The listing builds one solid part. Answer for the finished solid, in the listing's coordinates (mm). A direction names the side the tool comes from. Coordinates: 2 decimals unless noted, no trailing zeros. Loops run counter-clockwise (first coordinate to the right, second up) from the corner with the lowest first, then second, coordinate; pieces in that order, holes last. Notation, with made-up numbers: (-12.5, -31.5) - (16.5, -31.5) arc R31 ccw to (16.5, -5.5) - close; hole circle Ø7 at (78, -17). An arc over 180 degrees is marked (long way). Return JSON: item names as keys, results as strings. Group by question number.
1. Which of the six approach directions +Z, -Z, +X, -X, +Y, -Y give full straight-line access (tool end or side, diameter ignored) to faces 4 (the face through (0, 0.65, 1.4)), 5 (the face through (0.19, 7.45, 0.87)), 6 (the face through (-0.19, -7.49, 0.87))?
2. Each of these flat-tipped pins is pushed along its axis until it touches: P1, Ø1.5, axis at x = 1.5, y = 1, coming from the -Z side; P2, Ø1.6, axis at x = 0, z = 0, coming from the -Y side; P3, Ø1.1, axis at x = 0, z = 0, coming from the +Y side. Where does it stop, or does it pass through?
3. The mould has two halves that part along Y. Classify faces 1 (the face through (-1.2, 0.2, -1.6)), 2 (the face through (-1.024, 0.045, -0.472)), 3 (the face through (0.071, 2.575, 0.137)): pulls with the +Y half, pulls with the -Y half, needs draft (parallel to the pull), parting line crosses it, or undercut.
4. Find the intervals of material crossed by line 1 along Y through (x, z) = (0, -1.25) (3 decimals); line 2 along Y through (x, z) = (0.1, 1.6); line 3 along X through (y, z) = (0, -0.45) (3 decimals), in increasing order.
5. Section B-B (x = 1.45) is taken. Write down the section's boundary in (y, z).
6. Section C-C (y = 6.75) is taken. Write down the section's boundary in (x, z), and give its area (3 significant figures).
7. Section A-A (y = 1.5) is taken. Write down the section's boundary in (x, z), and give its area (3 significant figures).
```python
from build123d import *

# Parameters (mm, degrees)
SKETCH1_R                 = 2
BOSS_EXTRUDE1_DEPTH       = 12
SKETCH2_R                 = 1.025
CUT_EXTRUDE1_DEPTH        = 15.24
SKETCH3_W                 = 4
SKETCH3_H                 = 1.3
CUT_EXTRUDE2_DEPTH        = 15.24
F_2_56_TAPPED_HOLE1_D     = 1.778
F_2_56_TAPPED_HOLE1_DEPTH = 8.98398
F_2_56_TAPPED_HOLE1_TIP   = 0.53416509
F_2_56_TAPPED_HOLE2_D     = 1.778
F_2_56_TAPPED_HOLE2_DEPTH = 8.89
F_2_56_TAPPED_HOLE2_TIP   = 0.53416509


with BuildPart() as part:
    # Sketch1 → Boss-Extrude1 (new, symmetric)
    with BuildSketch(Plane(origin=(0, 0, 0), x_dir=(1, 0, 0), z_dir=(0, 1, 0))):
        with Locations(Location((0, 0, 0), (0, 0, 270))):
            Circle(SKETCH1_R)
    extrude(amount=BOSS_EXTRUDE1_DEPTH, both=True)

    # Sketch2 → Cut-Extrude1 (cut)
    with BuildSketch(Plane.XY.offset(1.016)):
        Circle(SKETCH2_R)
    extrude(amount=-CUT_EXTRUDE1_DEPTH, mode=Mode.SUBTRACT)

    # Sketch3 → Cut-Extrude2 (cut)
    with BuildSketch(Plane(origin=(0, 0, 1.016), x_dir=(-1, 0, 0), z_dir=(0, 0, -1))):
        Rectangle(SKETCH3_W, SKETCH3_H)
    extrude(amount=-CUT_EXTRUDE2_DEPTH, mode=Mode.SUBTRACT)

    # #2-56 Tapped Hole1
    with Locations(Plane(origin=(0, 12, 0), x_dir=(1, 0, 0), z_dir=(0, 1, 0))):
        with Locations((0, 0)):
            Hole(F_2_56_TAPPED_HOLE1_D / 2, depth=F_2_56_TAPPED_HOLE1_DEPTH)
            with Locations((0, 0, -(F_2_56_TAPPED_HOLE1_DEPTH + F_2_56_TAPPED_HOLE1_TIP / 2))):  # 118° drill point
                Cone(0, F_2_56_TAPPED_HOLE1_D / 2, F_2_56_TAPPED_HOLE1_TIP, mode=Mode.SUBTRACT)

    # #2-56 Tapped Hole2
    with Locations(Plane(origin=(0, -12, 0), x_dir=(-1, 0, 0), z_dir=(0, -1, 0))):
        with Locations((0, 0)):
            Hole(F_2_56_TAPPED_HOLE2_D / 2, depth=F_2_56_TAPPED_HOLE2_DEPTH)
            with Locations((0, 0, -(F_2_56_TAPPED_HOLE2_DEPTH + F_2_56_TAPPED_HOLE2_TIP / 2))):  # 118° drill point
                Cone(0, F_2_56_TAPPED_HOLE2_D / 2, F_2_56_TAPPED_HOLE2_TIP, mode=Mode.SUBTRACT)


solid = part.part
```
The answers:
{
 "1": {"face 4": "+Z, +X, -X", "face 5": "+Y", "face 6": "-Y"},
 "2": {"P1": "stops at z = -1.85", "P2": "stops at y = -3.06", "P3": "stops at y = 2.81"},
 "3": {"face 1": "needs draft", "face 2": "undercut", "face 3": "pulls with the +Y half"},
 "4": {"line 1": "y = -12 to -1.025, 1.025 to 12", "line 2": "y = -12 to -0.65, 0.65 to 12", "line 3": "x = -1.949 to -1.025, 1.025 to 1.949"},
 "5": {"outline": "(-12, -1.38) - (12, -1.38) - (12, 1.38) - (0.65, 1.38) - (0.65, 1.02) - (-0.65, 1.02) - (-0.65, 1.38) - (-12, 1.38) - close"},
 "6": {"outline": "circle Ø4 at (0, 0); hole circle Ø1.78 at (0, 0)", "area": "10.1 mm2"},
 "7": {"outline": "circle Ø4 at (0, 0)", "area": "12.6 mm2"}
}
